The listing builds one solid part. Answer for the finished solid, in the listing's coordinates (mm). A direction names the side the tool comes from. Give positions to 0.01 mm unless a question says otherwise; leave off trailing zeros. Write each loop counter-clockwise with the first axis right and the second up, starting at its lowest first coordinate (ties: lowest second). Pieces come first, ordered by that corner, then holes. Notation, with made-up numbers: (65, 79) -> (116, 79) arc R21 cw to (116, 88) -> close; hole circle Ø9 at (-26.75, 9.5). An arc over 180 degrees is marked (long way). Put each result on its own line as item: value. Start each with the question number.
1) A cutting plane is placed at A-A (y = -8). Give the number of separate pieces and of enclosed holes in the cut face, then the cut area to 3 significant figures.
2) A cutting plane is placed at C-C (z = 317.5). Write down the section's boundary in (x, y), then the cut area to 3 significant figures.
3) For faces 4 (the flat face through (0, 17.5, 394)), 5 (the flat face through (0, -15.9, 98)), determine the directions among +Z, -Z, +X, -X, +Y, -Y from which every point of the face is accessible in a straight line to the end or side of a thin tool.
4) For a pull along X with two mould halves and no side action, classify faces 1 (the flat face through (0, -15.9, 499)), 2 (the flat face through (0, -17.5, 499)), 3 (the flat face through (-17.5, 3, 394)) as released by +X, released by -X, zero draft, split by the parting line, or undercut.
5) Flat-ended cylindrical pins translate along their axes: pin 1 Ø1.3 at (x, y) = (2.5, -17) entering from -Z; pin 2 Ø1.3 at (x, y) = (-7, -17) entering from +Z; pin 3 Ø0.5 at (x, z) = (-17, 199.5) entering from -Y. Find the tip coordinate at first contact, or state that the pin passes through.
6) Find the intervals of material crossed by line 1 along Y through (x, z) = (-5, 543); line 2 along Y through (x, z) = (-15, 644), in increasing order. Write a range as from..to.
7) A cutting plane is placed at B-B (x = -3). Write down the section's boundary in (y, z).
Autodesk Inventor part; units mm, degrees
ref_plane "Start plane" through (0, 0, -17.5) normal (0, 0, 1) x (1, 0, 0)
ref_plane "End plane" through (0, 0, 817.5) normal (0, 0, 1) x (1, 0, 0)
ref_plane "Work Plane4" through (107.5, 0, -17.5) normal (0, 0, -1) x (-1, 0, 0)
ref_plane "Start plane" through (0, 0, -17.5) normal (0, 0, 1) x (1, 0, 0)
ref_plane "End plane" through (0, 0, 817.5) normal (0, 0, 1) x (1, 0, 0)
sketch "Sketch" plane through (0, 0, 0) normal (0, 0, 1) x (1, 0, 0)
  line L0 (-17.5, -14.3) -> (-17.5, 14.3)
  line L1 (-14.3, 17.5) -> (14.3, 17.5)
  line L2 (17.5, 14.3) -> (17.5, -14.3)
  line L3 (14.3, -17.5) -> (-14.3, -17.5)
  arc A0 (-17.5, -14.3) -> (-14.3, -17.5) centre (-14.3, -14.3) ccw
  arc A1 (-14.3, 17.5) -> (-17.5, 14.3) centre (-14.3, 14.3) ccw
  arc A2 (17.5, 14.3) -> (14.3, 17.5) centre (14.3, 14.3) ccw
  arc A3 (14.3, -17.5) -> (17.5, -14.3) centre (14.3, -14.3) ccw
  arc A4 (-14.3, 15.9) -> (-15.9, 14.3) centre (-14.3, 14.3) ccw
  line L4 (-14.3, 15.9) -> (14.3, 15.9)
  arc A5 (15.9, 14.3) -> (14.3, 15.9) centre (14.3, 14.3) ccw
  line L5 (15.9, 14.3) -> (15.9, -14.3)
  arc A6 (14.3, -15.9) -> (15.9, -14.3) centre (14.3, -14.3) ccw
  line L6 (14.3, -15.9) -> (-14.3, -15.9)
  arc A7 (-15.9, -14.3) -> (-14.3, -15.9) centre (-14.3, -14.3) ccw
  line L7 (-15.9, -14.3) -> (-15.9, 14.3)
  line L8 (0, 25.4278) -> (0, -25.4278) construction
  line L9 (-25.4278, 0) -> (25.4278, 0) construction
  dimension "d7" = 3.2
  dimension "d10" = 35
  dimension "d11" = 35
  dimension "d12" = 1.6
  dimension "d15" = 17.5
  dimension "d16" = 17.5
extrude "Body" add sketch "Sketch" along normal up to surface (835 mm away) from surface at -17.5
sketch "Sketch3" plane through (0, 0, 0) normal (0, 0, 1) x (1, 0, 0)
  line L0 (0, 0) -> (10, 0)
ref_plane "Work Plane3" through (0, 0, 0) normal (0, -1, 0) x (1, 0, 0)
sketch "Sketch4" plane through (0, 0, 0) normal (0, -1, 0) x (1, 0, 0)
  line L0 (-2, -17.5) -> (12, -17.5)
  line L1 (-2, 817.5) -> (12, 817.5)
  dimension "d18" = 835
ref_plane "Work Plane4" through (107.5, 0, -17.5) normal (0, 0, -1) x (-1, 0, 0)
split "Split1" plane through (107.5, 0, -17.5) removes the side toward (0, 0, -1)
ref_plane "Work Plane5" through (17.5, 0, 817.5) normal (0, 0, 1) x (1, 0, 0)
split "Split2" plane through (17.5, 0, 817.5) removes the side toward (0, 0, 1)
ref_plane "Work Plane6" through (0, 17.5, -17.5) normal (0, -0.7071, -0.7071) x (1, 0, 0)
split "Split3" plane through (0, 17.5, -17.5) removes the side toward (0, -0.7071, -0.7071)
ref_plane "Work Plane14" through (0, 17.5, 817.5) normal (0, -0.7071, 0.7071) x (1, 0, 0)
split "Split5" plane through (0, 17.5, 817.5) removes the side toward (0, -0.7071, 0.7071)
ref_plane "Work Plane17" through (0, 0, 200) normal (0, -1, 0) x (0, 0, -1)
ref_plane "Work Plane18" through (0, -500, 200) normal (0, -1, 0) x (0, 0, -1)
ref_plane "Work Plane19" through (0, -250, 200) normal (0, -1, 0) x (0, 0, -1)
sketch "Sketch17" plane through (0, -250, 200) normal (0, -1, 0) x (0, 0, -1)
  arc A0 (-17.5, -14.3) -> (-14.3, -17.5) centre (-14.3, -14.3) ccw
  line L0 (-17.5, -14.3) -> (-17.5, 14.3)
  arc A1 (-14.3, 17.5) -> (-17.5, 14.3) centre (-14.3, 14.3) ccw
  line L1 (-14.3, 17.5) -> (14.3, 17.5)
  arc A2 (17.5, 14.3) -> (14.3, 17.5) centre (14.3, 14.3) ccw
  line L2 (17.5, 14.3) -> (17.5, -14.3)
  arc A3 (14.3, -17.5) -> (17.5, -14.3) centre (14.3, -14.3) ccw
  line L3 (14.3, -17.5) -> (-14.3, -17.5)
  arc A4 (-14.3, 15.9) -> (-15.9, 14.3) centre (-14.3, 14.3) ccw
  line L4 (-14.3, 15.9) -> (14.3, 15.9)
  arc A5 (15.9, 14.3) -> (14.3, 15.9) centre (14.3, 14.3) ccw
  line L5 (15.9, 14.3) -> (15.9, -14.3)
  arc A6 (14.3, -15.9) -> (15.9, -14.3) centre (14.3, -14.3) ccw
  line L6 (14.3, -15.9) -> (-14.3, -15.9)
  arc A7 (-15.9, -14.3) -> (-14.3, -15.9) centre (-14.3, -14.3) ccw
  line L7 (-15.9, -14.3) -> (-15.9, 14.3)
extrude "Extrusion14" cut sketch "Sketch17" along normal up to surface (500 mm away) from surface at -250 contours L0 A1 L1 A2 L2 A3 L3 A0 | L4 A5 L5 A6 L6 A7 L7 A4
ref_plane "Work Plane20" through (0, 0, 400) normal (0, -1, 0) x (0, 0, -1)
ref_plane "Work Plane21" through (0, -500, 400) normal (0, -1, 0) x (0, 0, -1)
ref_plane "Work Plane22" through (0, -250, 400) normal (0, -1, 0) x (0, 0, -1)
sketch "Sketch18" plane through (0, -250, 400) normal (0, -1, 0) x (0, 0, -1)
  arc A0 (-17.5, -14.3) -> (-14.3, -17.5) centre (-14.3, -14.3) ccw
  line L0 (-17.5, -14.3) -> (-17.5, 14.3)
  arc A1 (-14.3, 17.5) -> (-17.5, 14.3) centre (-14.3, 14.3) ccw
  line L1 (-14.3, 17.5) -> (14.3, 17.5)
  arc A2 (17.5, 14.3) -> (14.3, 17.5) centre (14.3, 14.3) ccw
  line L2 (17.5, 14.3) -> (17.5, -14.3)
  arc A3 (14.3, -17.5) -> (17.5, -14.3) centre (14.3, -14.3) ccw
  line L3 (14.3, -17.5) -> (-14.3, -17.5)
  arc A4 (-14.3, 15.9) -> (-15.9, 14.3) centre (-14.3, 14.3) ccw
  line L4 (-14.3, 15.9) -> (14.3, 15.9)
  arc A5 (15.9, 14.3) -> (14.3, 15.9) centre (14.3, 14.3) ccw
  line L5 (15.9, 14.3) -> (15.9, -14.3)
  arc A6 (14.3, -15.9) -> (15.9, -14.3) centre (14.3, -14.3) ccw
  line L6 (14.3, -15.9) -> (-14.3, -15.9)
  arc A7 (-15.9, -14.3) -> (-14.3, -15.9) centre (-14.3, -14.3) ccw
  line L7 (-15.9, -14.3) -> (-15.9, 14.3)
extrude "Extrusion15" cut sketch "Sketch18" along normal up to surface (500 mm away) from surface at -250 contours L0 A1 L1 A2 L2 A3 L3 A0 | L4 A5 L5 A6 L6 A7 L7 A4
ref_plane "Work Plane23" through (0, 0, 600) normal (0, -1, 0) x (0, 0, -1)
ref_plane "Work Plane24" through (0, -500, 600) normal (0, -1, 0) x (0, 0, -1)
ref_plane "Work Plane25" through (0, -250, 600) normal (0, -1, 0) x (0, 0, -1)
sketch "Sketch19" plane through (0, -250, 600) normal (0, -1, 0) x (0, 0, -1)
  arc A0 (-17.5, -14.3) -> (-14.3, -17.5) centre (-14.3, -14.3) ccw
  line L0 (-17.5, -14.3) -> (-17.5, 14.3)
  arc A1 (-14.3, 17.5) -> (-17.5, 14.3) centre (-14.3, 14.3) ccw
  line L1 (-14.3, 17.5) -> (14.3, 17.5)
  arc A2 (17.5, 14.3) -> (14.3, 17.5) centre (14.3, 14.3) ccw
  line L2 (17.5, 14.3) -> (17.5, -14.3)
  arc A3 (14.3, -17.5) -> (17.5, -14.3) centre (14.3, -14.3) ccw
  line L3 (14.3, -17.5) -> (-14.3, -17.5)
  arc A4 (-14.3, 15.9) -> (-15.9, 14.3) centre (-14.3, 14.3) ccw
  line L4 (-14.3, 15.9) -> (14.3, 15.9)
  arc A5 (15.9, 14.3) -> (14.3, 15.9) centre (14.3, 14.3) ccw
  line L5 (15.9, 14.3) -> (15.9, -14.3)
  arc A6 (14.3, -15.9) -> (15.9, -14.3) centre (14.3, -14.3) ccw
  line L6 (14.3, -15.9) -> (-14.3, -15.9)
  arc A7 (-15.9, -14.3) -> (-14.3, -15.9) centre (-14.3, -14.3) ccw
  line L7 (-15.9, -14.3) -> (-15.9, 14.3)
extrude "Extrusion16" cut sketch "Sketch19" along normal up to surface (500 mm away) from surface at -250 contours L0 A1 L1 A2 L2 A3 L3 A0 | L4 A5 L5 A6 L6 A7 L7 A4
equation "\"d7\" = G_IR"
equation "\"d10\" = G_H"
equation "\"d11\" = G_W"
equation "\"d12\" = G_T"
equation "\"d15\" = 0.5 * d10"
equation "\"d16\" = 0.5 * d11"
equation "\"d3\" = G_L"
equation "\"G_W\" = 35"
equation "\"G_H\" = 35"
equation "\"G_T\" = 1.6"
equation "\"G_IR\" = 3.2"
equation "\"G_L\" = 835"
equation "\"G_OFFSET_START\" = 17.5"
equation "\"G_OFFSET_END\" = 17.5"
equation "\"d13\" = -G_OFFSET_START"
equation "\"d14\" = G_OFFSET_END + B_L"
properties part number "AS 1163 - C350L0 35x35x1.6 SHS - 835" material "Steel, Mild"
Reply:
1. separate pieces: 8
1. enclosed holes: 0
1. area: 2,200 mm2
2. outline: (-17.5, -14.3) arc R3.2 ccw to (-14.3, -17.5) -> (14.3, -17.5) arc R3.2 ccw to (17.5, -14.3) -> (17.5, 14.3) arc R3.2 ccw to (14.3, 17.5) -> (-14.3, 17.5) arc R3.2 ccw to (-17.5, 14.3) -> close; hole (-15.9, -14.3) arc R1.6 ccw to (-14.3, -15.9) -> (14.3, -15.9) arc R1.6 ccw to (15.9, -14.3) -> (15.9, 14.3) arc R1.6 ccw to (14.3, 15.9) -> (-14.3, 15.9) arc R1.6 ccw to (-15.9, 14.3) -> close
2. area: 207 mm2
3. face 4: +Z, -Z, +X, -X, +Y
3. face 5: +Z, -Z
4. face 1: undercut
4. face 2: zero draft
4. face 3: released by -X
5. pin 1: stops at z = 16.35
5. pin 2: stops at z = 783.65
5. pin 3: stops at y = 0
6. line 1: y = -17.5..-15.9, 15.9..17.5
6. line 2: y = -17.42..-15.74, 15.74..17.42
7. outline: (-17.5, 17.5) -> (-15.9, 15.9) -> (-15.9, 182.5) -> (-17.5, 182.5) -> close; (-17.5, 217.5) -> (-15.9, 217.5) -> (-15.9, 382.5) -> (-17.5, 382.5) -> close; (-17.5, 417.5) -> (-15.9, 417.5) -> (-15.9, 582.5) -> (-17.5, 582.5) -> close; (-17.5, 617.5) -> (-15.9, 617.5) -> (-15.9, 784.1) -> (-17.5, 782.5) -> close; (15.9, -15.9) -> (17.5, -17.5) -> (17.5, 817.5) -> (15.9, 815.9) -> close
